Autodesk Fusion 360 part; units mm, degrees
sketch "Sketch1" plane through (0, 0, 0) normal (0, 0, 1) x (1, 0, 0)
  circle A0 centre (0, 0) radius 50
extrude "Extrude1" add sketch "Sketch1" along normal blind 20
ref_plane "WorkPlane1" through (0, 0, 10) normal (0, 0, 1) x (1, 0, 0)
sketch "Sketch2" plane through (0, 0, 10) normal (0, 0, 1) x (1, 0, 0)
  circle A0 centre (0, 0) radius 47.5
extrude "Extrude2" cut sketch "Sketch2" along normal blind 10
sketch "Sketch3" plane through (0, 0, 0) normal (0, 0, 1) x (1, 0, 0)
  circle A0 centre (0, 0) radius 20
extrude "Extrude3" add sketch "Sketch3" against normal blind 20
sketch "Sketch4" plane through (0, 0, -20) normal (0, 0, -1) x (1, 0, 0)
  circle A0 centre (0, 0) radius 20
shell "Shell1" thickness 1 outward yes removed faces 1 at (6.3705, -1.965, -20)
sketch "Sketch5" plane through (0, 0, 10) normal (0, 0, 1) x (1, 0, 0)
  line L0 (0, 0) -> (20, 0)
  line L1 (0, 0) -> (0, 20)
  line L2 (0, 0) -> (-20, 0)
  line L3 (0, 0) -> (0, -20)
  line L4 (-10, 20) -> (12.1822, 20)
  line L5 (-10, -20) -> (12.7429, -20)
  line L6 (-20, 10) -> (-20, -10)
  line L7 (20, 10) -> (20, -10)
ref_plane "WorkPlane2" through (-20, 0, 10) normal (-0.7071, 0, 0.7071) x (0, -1, 0)
sketch "Sketch6" plane through (-20, 0, 10) normal (-0.7071, 0, 0.7071) x (0, -1, 0)
  circle A0 centre (0, 0) radius 5
  dimension "d17" = 10
extrude "Extrude4" cut sketch "Sketch6" against normal blind 10
ref_plane "WorkPlane3" through (1.3715, -20, 10) normal (0, -0.7071, 0.7071) x (1, 0, 0)
sketch "Sketch7" plane through (0, 0, 10) normal (0, 0, 1) x (1, 0, 0)
sketch "Sketch8" plane through (1.3715, -20, 10) normal (0, -0.7071, 0.7071) x (1, 0, 0)
  circle A0 centre (0, 0) radius 5
  dimension "d21" = 10
extrude "Extrude5" cut sketch "Sketch8" against normal blind 30
ref_plane "WorkPlane4" through (20, 0, 10) normal (0.7071, 0, 0.7071) x (0, -1, 0)
sketch "Sketch9" plane through (20, 0, 10) normal (0.7071, 0, 0.7071) x (0, -1, 0)
  circle A0 centre (0, 0) radius 5
  dimension "d25" = 10
ref_plane "WorkPlane5" through (1.0911, 20, 10) normal (0, 0.7071, 0.7071) x (1, 0, 0)
sketch "Sketch10" plane through (1.0911, 20, 10) normal (0, 0.7071, 0.7071) x (1, 0, 0)
  circle A0 centre (0, 0) radius 5
  dimension "d27" = 10
extrude "Extrude6" cut sketch "Sketch9" against normal blind 20
extrude "Extrude7" cut sketch "Sketch10" against normal blind 10
Source: CAD feature listing. Evaluate the final solid. Frame: model axes, mm. A direction names the side the tool comes from. Coordinates: 2 decimals unless noted, no trailing zeros. Loops run counter-clockwise (first coordinate to the right, second up) from the corner with the lowest first, then second, coordinate; pieces in that order, holes last. Notation, with made-up numbers: (-2.5, 47) - (51.5, 47) arc R18 ccw to (51.5, 76) - close; hole circle Ø5 at (79.5, 61.5). An arc over 180 degrees is marked (long way). One line per question, with ' | ' between items.
1) Set-up query: faces 5 (the face through (-4.336, -19.524, -9.86)), 6 (the face through (-1, 1, 10)), 7 (the face through (41.3, -22.4, 21)), 8 (the face through (-1, 1, 11)). Return all of +Z, -Z, +X, -X, +Y, -Y with unobstructed straight access to the full face (end or side cutting, diameter ignored); none if empty.
Report:
face 5: -Z | face 6: none | face 7: +Z, +X, -X, +Y, -Y | face 8: +Z
2) First-contact query: P1, Ø3, axis at x = -39, z = 10.5, coming from the +Y side; P2, Ø1.5, axis at x = -12.5, z = 7.5, coming from the +Y side; P3, Ø1.5, axis at y = -1, z = 9, coming from the -X side. Flat tips, straight axial feed; report the tip coordinate or a pass-through.
Report:
P1: stops at y = 34.57 | P2: stops at y = 49.63 | P3: stops at x = -51
3) Section C-C, the plane x = 0. Give the number of separate pieces and of enclosed holes in the cut face, then the cut area to 3 significant figures.
Report:
separate pieces: 3 | enclosed holes: 0 | area: 250 mm²
4) Line query: line 1 along Y through (x, z) = (0, 14); line 2 along Z through (x, y) = (17.5, 46.5); line 3 along X through (y, z) = (-39, 18.5). Output: solid intervals per line, ascending.
Report:
line 1: y = -51 to -50, -47.5 to -46.5, 46.5 to 47.5, 50 to 51 | line 2: z = -1 to 0, 20 to 21 | line 3: x = -32.86 to -31.29, -27.12 to -25.32, 25.32 to 27.12, 31.29 to 32.86
5) Section B-B, the plane y = 35.5. Return loops of the section in (x, z).
Report:
outline: (-36.62, -1) - (36.62, -1) - (36.62, 21) - (30.03, 21) - (30.03, 11) - (-30.03, 11) - (-30.03, 21) - (-36.62, 21) - close; hole (-35.21, 0) - (35.21, 0) - (35.21, 20) - (31.56, 20) - (31.56, 10) - (-31.56, 10) - (-31.56, 20) - (-35.21, 20) - close
6) Section D-D, the plane z = -13. Return loops of the section in (x, y), then the cut area to 3 significant figures.
Report:
outline: circle Ø42 at (0, 0); hole circle Ø40 at (0, 0) | area: 129 mm²
7) Section A-A, the plane x = -31. Return loops of the section in (y, z).
Report:
outline: (-40.5, -1) - (40.5, -1) - (40.5, 21) - (34.66, 21) - (34.66, 11) - (-34.66, 11) - (-34.66, 21) - (-40.5, 21) - close; hole (-39.23, 0) - (39.23, 0) - (39.23, 20) - (35.99, 20) - (35.99, 10) - (-35.99, 10) - (-35.99, 20) - (-39.23, 20) - close
8) Pull-direction query (Z, two-part tool) for faces 1 (the face through (22, 1, -1)), 2 (the face through (-11.056, 49.787, 9.846)), 3 (the face through (44.2, -18.3, 20)), 4 (the face through (-10.3, 46.37, 14.93)); classes: released by +Z, released by -Z, zero draft, split by the parting line, or undercut.
Report:
face 1: released by -Z | face 2: zero draft | face 3: undercut | face 4: undercut
